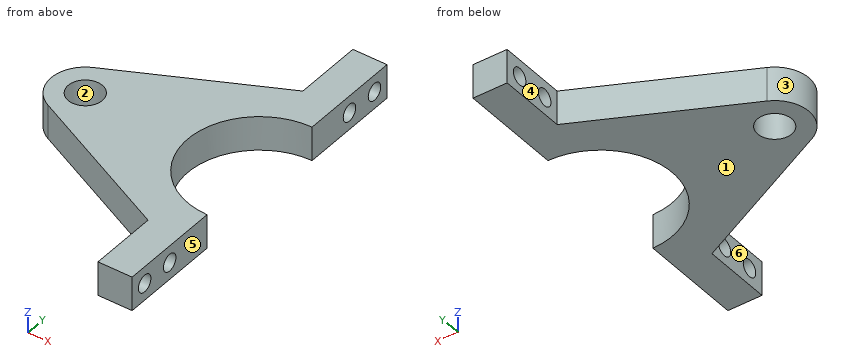
from build123d import *

# Parameters (mm, degrees)
BOSS_EXTRUDE1_DEPTH = 10
SKETCH2_R           = 5
CUT_EXTRUDE1_DEPTH  = 83.27950738
SKETCH3_R           = 2.5
CUT_EXTRUDE2_DEPTH  = 76.159549646


with BuildPart() as part:
    # Sketch1 → Boss-Extrude1 (new body)
    with BuildSketch(Plane.XY):
        with BuildLine():
            Line((0, 24.299679487), (0, 54.25))
            Line((0, 54.25), (-10, 54.25))
            Line((-10, 54.25), (-10, 34.25))
            Line((-10, 34.25), (-55.400247003, 12.302884399))
            ThreePointArc((-55.400247003, 12.302884399), (-61.047971586, 3.299679487), (-55.400247003, -5.703525425))
            Line((-55.400247003, -5.703525425), (-10, -27.650641026))
            Line((-10, -27.650641026), (-10, -47.650641026))
            Line((-10, -47.650641026), (0, -47.650641026))
            Line((0, -47.650641026), (0, -17.700320513))
            ThreePointArc((0, -17.700320513), (-21, 3.299679487), (0, 24.299679487))
        make_face()
    extrude(amount=-BOSS_EXTRUDE1_DEPTH)

    # Sketch2 → Cut-Extrude1 (cut, through all)
    with BuildSketch(Plane.XY):
        with Locations((-51.047971586, 3.299679487)):
            Circle(SKETCH2_R)
    extrude(amount=-CUT_EXTRUDE1_DEPTH, mode=Mode.SUBTRACT)

    # Sketch3 → Cut-Extrude2 (cut, through all)
    with BuildSketch(Plane.ZY.offset(10)):
        with Locations((-5, 49.25)):
            Circle(SKETCH3_R)
        with Locations((-5, 39.25)):
            Circle(SKETCH3_R)
        with Locations(Location((-5, -32.650641026, 0), (0, 0, 180))):
            Circle(SKETCH3_R)
        with Locations(Location((-5, -42.650641026, 0), (0, 0, 180))):
            Circle(SKETCH3_R)
    extrude(amount=-CUT_EXTRUDE2_DEPTH, mode=Mode.SUBTRACT)


solid = part.part
CAD build for the part. Positions are in the model's coordinates, mm. Face numbers are marked on the shaded views. A direction names the side the tool comes from. Coordinates: 2 decimals unless noted, no trailing zeros. Write each loop counter-clockwise with the first axis right and the second up, starting at its lowest first coordinate (ties: lowest second). Pieces come first, ordered by that corner, then holes. Notation, with made-up numbers: M 4.25,40.5 L 42.25,40.5 A18 cw 42.25,58.5 Z; hole C 71.5,-32 d7. An arc over 180 degrees is marked long. Answer as a JSON object with one key per item and string values. Group by question number.
1) Tool access for the marked faces 4, 5 and 6: list every direction of +Z, -Z, +X, -X, +Y, -Y with a clear straight run to the whole face (end or side of a thin tool).
2) Saw through at A-A (y = 49.25). Write the cut outline in (x, z).
3) Mould opens along Y. For the marked faces 1, 2 and 3 say: +Y half, -Y half, draft (parallel to the pull), parting line (faces both ways), or undercut.
4) Saw through at C-C (x = -50.5). Write the cut outline in (y, z).
5) Saw through at B-B (z = -4.25). Write the cut outline in (x, y).
6) Pin check, flat tips, straight feed: pin 1 Ø4.5 at (y, z) = (-42.65, -5) entering from -X; pin 2 Ø1 at (y, z) = (-23.5, -2.5) entering from -X; pin 3 Ø1.5 at (y, z) = (-26, -2) entering from -X; pin 4 Ø5 at (y, z) = (13, -6.5) entering from -X. Stop position of each tip, or through.
7) Wall check: line 1 (Y direction, x = -8.5, z = -4); line 2 (Y direction, x = -5.5, z = -5); line 3 (Y direction, x = -47.5, z = -8.75). Give the ranges that are in metal, low to high. Write a range as from..to.
8) Saw through at D-D (z = -8.75). Write the cut outline in (x, y), plus the area to 3 significant figures.
Values follow:
{
 "1": {"face 4": "+Z, -Z, -X, +Y", "face 5": "+Z, -Z, +X, +Y, -Y", "face 6": "+Z, -Z, -X, -Y"},
 "2": {"outline": "M -10,-10 L 0,-10 L 0,-7.5 L -10,-7.5 Z; M -10,-2.5 L 0,-2.5 L 0,0 L -10,0 Z"},
 "3": {"face 1": "draft", "face 2": "undercut", "face 3": "parting line"},
 "4": {"outline": "M -8.07,-10 L -1.67,-10 L -1.67,0 L -8.07,0 Z; M 8.27,-10 L 14.67,-10 L 14.67,0 L 8.27,0 Z"},
 "5": {"outline": "M -55.4,-5.7 L -10,-27.65 L -10,-30.27 L 0,-30.27 L 0,-17.7 A21 cw 0,24.3 L 0,36.87 L -10,36.87 L -10,34.25 L -55.4,12.3 A10 ccw Z; M -10,-47.65 L 0,-47.65 L 0,-45.04 L -10,-45.04 Z; M -10,-40.27 L 0,-40.27 L 0,-35.04 L -10,-35.04 Z; M -10,41.63 L 0,41.63 L 0,46.87 L -10,46.87 Z; M -10,51.63 L 0,51.63 L 0,54.25 L -10,54.25 Z; hole C -51.05,3.3 d10"},
 "6": {"pin 1": "passes through", "pin 2": "stops at x = -19.62", "pin 3": "stops at x = -14.97", "pin 4": "stops at x = -57.99"},
 "7": {"line 1": "y = -47.65..-44.94, -40.36..-34.94, -30.36..-15.9, 22.5..36.96, 41.54..46.96, 51.54..54.25", "line 2": "y = -47.65..-45.15, -40.15..-35.15, -30.15..-16.97, 23.57..36.75, 41.75..46.75, 51.75..54.25", "line 3": "y = -9.52..-0.22, 6.82..16.12"},
 "8": {"outline": "M -55.4,-5.7 L -10,-27.65 L -10,-47.65 L 0,-47.65 L 0,-17.7 A21 cw 0,24.3 L 0,54.25 L -10,54.25 L -10,34.25 L -55.4,12.3 A10 ccw Z; hole C -51.05,3.3 d10", "area": "2,130 mm2"}
}
